from build123d import *

# Parameters (mm, degrees)
F0_W      = 76.2
F0_H      = 120.65
F1_DEPTH  = 6.35
F2_W      = 12.7
F2_H      = 25.4
F3_DEPTH  = 6.35
F4_R      = 2.54
F5_DEPTH  = 6.35
F6_W      = 12.7
F6_H      = 2.54
F7_DEPTH  = 2.54
F8_R      = 0.762
F9_R      = 0.762
F10_DEPTH = 11.938
F11_W     = 66.04
F11_H     = 110.49
F12_DEPTH = 3.81


with BuildPart() as f1:
    # F0 (on Top) → F1 (new body)
    with BuildSketch(Plane.XY):
        with Locations((-0.644507, -3.87145)):
            Rectangle(F0_W, F0_H)
    extrude(amount=F1_DEPTH)

    # F2 (on face) → F3 (cut)
    with BuildSketch(Plane.XY.offset(6.35)):
        Rectangle(F2_W, F2_H)
    extrude(amount=-F3_DEPTH, mode=Mode.SUBTRACT)

    # F4 (on face) → F5 (cut)
    with BuildSketch(Plane.XY.offset(6.35)):
        with Locations((0, -32.7025)):
            Circle(F4_R)
        with Locations((0, 32.7025)):
            Circle(F4_R)
    extrude(amount=-F5_DEPTH, mode=Mode.SUBTRACT)

    # F6 (on face) → F7 (join)
    with BuildSketch(Plane.XY.offset(6.35)):
        with Locations((-13.97, 11.43)):
            Rectangle(F6_W, F6_H)
        with Locations((-13.97, -11.43)):
            Rectangle(F6_W, F6_H)
    extrude(amount=F7_DEPTH)

    # F8 (on face) + F9 (on face) → F10 (cut)
    with BuildSketch(Plane.XY.offset(8.89)):
        with Locations((-13.97, 11.43)):
            Circle(F8_R)
    with BuildSketch(Plane.XY.offset(8.89)):
        with Locations((-13.97, -11.43)):
            Circle(F9_R)
    extrude(amount=-F10_DEPTH, mode=Mode.SUBTRACT)

    # F11 (on face) → F12 (cut)
    with BuildSketch(Plane(origin=(0, 0, 0), x_dir=(1, 0, 0), z_dir=(0, 0, -1))):
        with Locations((-0.644507, 3.87145)):
            Rectangle(F11_W, F11_H)
    extrude(amount=-F12_DEPTH, mode=Mode.SUBTRACT)


solid = f1.part
CAD build for the part. Positions are in the model's coordinates, mm. A direction names the side the tool comes from. Coordinates: 2 decimals unless noted, no trailing zeros. Order: outer loops, then holes, each group sorted by start corner. A loop starts at its lowest first (then second) coordinate and runs counter-clockwise, first axis right, second up.
Item 1: Pin check, flat tips, straight feed: pin 1 Ø2 at (y, z) = (-11, 8) entering from +X; pin 2 Ø1.5 at (y, z) = (2.5, 7.5) entering from -X; pin 3 Ø6 at (x, y) = (0, 32.7) entering from -Z; pin 4 Ø0.8 at (y, z) = (11, 8) entering from -X. Stop position of each tip, or through.
Check sheet entries:
pin 1: stops at x = -7.62
pin 2: passes through
pin 3: stops at z = 3.81
pin 4: stops at x = -20.32
Item 2: Band-saw the part on A-A on x = -5. List the corners of the cut face in (y, z), plus the area to 3 significant figures.
Check sheet entries:
outline: (-64.2, 0) - (-59.12, 0) - (-59.12, 3.81) - (-12.7, 3.81) - (-12.7, 6.35) - (-64.2, 6.35) - close; (12.7, 3.81) - (51.37, 3.81) - (51.37, 0) - (56.45, 0) - (56.45, 6.35) - (12.7, 6.35) - close
area: 281 mm2
Item 3: Drill centre lines: L1, parallel to Y at x = -13.97, z = 7.15; L2, parallel to Y at x = -13.97, z = 5.15; L3, parallel to X at y = -4, z = 3. Where is each one in solid material? Low to high.
Check sheet entries:
L1: y = -12.7 to -12.19, -10.67 to -10.16, 10.16 to 10.67, 12.19 to 12.7
L2: y = -64.2 to -12.19, -10.67 to 10.67, 12.19 to 56.45
L3: x = -38.74 to -33.66, 32.38 to 37.46
Item 4: Two-plate mould, pull along X, no slides. Class faces 4 (the face through (-7.62, 11, 8)), 5 (the face through (-35, 1, 0)), 6 (the face through (0, -12.7, 5)): +X half, -X half, draft (parallel to the pull), parting line (faces both ways), or undercut.
Check sheet entries:
face 4: +X half
face 5: draft
face 6: undercut
Item 5: 3-axis set-ups, long thin cutter, end or side, ignore diameter. For faces 1 (the face through (-20.32, 11, 8)), 2 (the face through (-6.35, 0, 5)), 3 (the face through (-14, 12.7, 8)): which of +Z, -Z, +X, -X, +Y, -Y reach the whole face in a straight line?
Check sheet entries:
face 1: +Z, -X, +Y, -Y
face 2: +Z, -Z
face 3: +Z, +X, -X, +Y
Item 6: Band-saw the part on B-B on y = 0. List the corners of the cut face in (x, z), plus the area to 3 significant figures.
Check sheet entries:
outline: (-38.74, 0) - (-33.66, 0) - (-33.66, 3.81) - (-6.35, 3.81) - (-6.35, 6.35) - (-38.74, 6.35) - close; (6.35, 3.81) - (32.38, 3.81) - (32.38, 0) - (37.46, 0) - (37.46, 6.35) - (6.35, 6.35) - close
area: 200 mm2
Item 7: Band-saw the part on C-C on z = 1.5. List the corners of the cut face in (x, y).
Check sheet entries:
outline: (-38.74, -64.2) - (37.46, -64.2) - (37.46, 56.45) - (-38.74, 56.45) - close; hole (-33.66, -59.12) - (32.38, -59.12) - (32.38, 51.37) - (-33.66, 51.37) - close
Item 8: Band-saw the part on D-D on y = 48.5. List the corners of the cut face in (x, z), plus the area to 3 significant figures.
Check sheet entries:
outline: (-38.74, 0) - (-33.66, 0) - (-33.66, 3.81) - (32.38, 3.81) - (32.38, 0) - (37.46, 0) - (37.46, 6.35) - (-38.74, 6.35) - close
area: 232 mm2
